Model file for the job. Use its own axes, mm. A direction names the side the tool comes from. Round coordinates to 2 decimals unless told otherwise and drop trailing zeros. Loops run counter-clockwise (first coordinate to the right, second up) from the corner with the lowest first, then second, coordinate; pieces in that order, holes last. Notation, with made-up numbers: M 55,51 L 98,51 A14 ccw 98,69 Z; hole C 17.25,67 d10. An arc over 180 degrees is marked long. Answer in a Markdown table with one row per item.
from build123d import *

# Parameters (mm, degrees)
SKETCH1_W                  = 10
SKETCH1_H                  = 9.1
BASE_FLANGE1_DEPTH         = 0.3
TAB1_DEPTH                 = 0.3
SKETCHED_START             = -12
SKETCHED_BEND1_OUTLINE_W   = 2.75
SKETCHED_BEND1_OUTLINE_H   = 0.3
SKETCHED_BEND1_DEPTH       = 6.725504
SKETCHED_START_2           = -5.274496
SKETCHED_BEND1_2_OUTLINE_W = 2.75
SKETCHED_BEND1_2_OUTLINE_H = 0.3
SKETCHED_BEND1_2_DEPTH     = 0.074434719
SKETCHED_START_3           = -5.35
SKETCHED_BEND1_3_DEPTH     = 0.8
SKETCHED_START_4           = -1.375
SKETCHED_BEND1_4_DEPTH     = 2.75
FILLET1_R                  = 1.5
SKETCH13_R                 = 0.8
CUT_EXTRUDE2_DEPTH         = 13.370499101


with BuildPart() as part:
    # Base-Flange1: sheet metal written as solids
    # Sketch1 → Base-Flange1 (new body)
    with BuildSketch(Plane.XY):
        Rectangle(SKETCH1_W, SKETCH1_H)
    extrude(amount=BASE_FLANGE1_DEPTH)

    # Tab1: sheet metal written as solids
    # Sketch7 → Tab1 (add)
    with BuildSketch(Plane.XY):
        with BuildLine():
            Line((1.375, 0), (1.375, -9.175))
            ThreePointArc((1.375, -9.175), (0, -10.55), (-1.375, -9.175))
            Line((-1.375, -9.175), (-1.375, 0))
            ThreePointArc((-1.375, 0), (0, 1.375), (1.375, 0))
        make_face()
    extrude(amount=TAB1_DEPTH)

    # Sketched Bend1: read off the stored shape, not the designer's step
    # Sketched Bend1 outline → Sketched Bend1 (cut)
    with BuildSketch(Plane(origin=(0, 0, 0), x_dir=(1, 0, 0), z_dir=(0, 1, 0)).offset(SKETCHED_START)):
        with Locations((0, -0.15)):
            Rectangle(SKETCHED_BEND1_OUTLINE_W, SKETCHED_BEND1_OUTLINE_H)
    extrude(amount=SKETCHED_BEND1_DEPTH, mode=Mode.SUBTRACT)

    # Sketched Bend1 2 outline → Sketched Bend1 2 (cut)
    with BuildSketch(Plane(origin=(0, 0, 0), x_dir=(1, 0, 0), z_dir=(0, 1, 0)).offset(SKETCHED_START_2)):
        with Locations((0, -0.15)):
            Rectangle(SKETCHED_BEND1_2_OUTLINE_W, SKETCHED_BEND1_2_OUTLINE_H)
    extrude(amount=SKETCHED_BEND1_2_DEPTH, mode=Mode.SUBTRACT)

    # Sketched Bend1 3 outline → Sketched Bend1 3 (add)
    with BuildSketch(Plane(origin=(0, 0, 0), x_dir=(1, 0, 0), z_dir=(0, 1, 0)).offset(SKETCHED_START_3)):
        with BuildLine():
            Line((-1.375, 4.103982388), (-1.375, 0))
            Line((-1.375, 0), (1.375, 0))
            Line((1.375, 0), (1.375, 4.103982388))
            ThreePointArc((1.375, 4.103982388), (0, 5.478982388), (-1.375, 4.103982388))
        make_face()
    extrude(amount=SKETCHED_BEND1_3_DEPTH)

    # Sketched Bend1 4 outline → Sketched Bend1 4 (cut)
    with BuildSketch(Plane.YZ.offset(SKETCHED_START_4)):
        with BuildLine():
            Line((-5.05, -0.5), (-5.05, -7))
            Line((-5.05, -7), (-4.55, -7))
            Line((-4.55, -7), (-4.55, 0))
            ThreePointArc((-4.55, 0), (-4.903553391, -0.146446609), (-5.05, -0.5))
        make_face()
        with BuildLine():
            Line((-7, -7), (-5.349999999, -7))
            Line((-5.349999999, -7), (-5.35, -0.5))
            ThreePointArc((-5.35, -0.5), (-5.115685425, 0.065685425), (-4.55, 0.3))
            Line((-4.55, 0.3), (-3, 0.3))
            Line((-3, 0.3), (-3, 2))
            Line((-3, 2), (-5.200061281, 2))
            Line((-5.200061281, 2), (-5.200061281, 0))
            Line((-5.200061281, 0), (-7, 0))
            Line((-7, 0), (-7, -7))
        make_face()
    extrude(amount=SKETCHED_BEND1_4_DEPTH, mode=Mode.SUBTRACT)

    # Fillet1
    fillet1_edges = [part.edges().sort_by_distance(p)[0] for p in [
        (-5, 4.55, 0.15),
        (5, 4.55, 0.15),
        (5, -4.55, 0.15),
        (-5, -4.55, 0.15),
    ]]
    fillet(fillet1_edges, radius=FILLET1_R)

    # Sketch13 → Cut-Extrude2 (cut, through all)
    with BuildSketch(Plane.XZ.offset(5.35)):
        with Locations(Location((0, -4.103982388, 0), (0, 0, 270))):
            Circle(SKETCH13_R)
    extrude(amount=-CUT_EXTRUDE2_DEPTH, mode=Mode.SUBTRACT)

    # Sketch14 → Revolve1 (revolve)
    with BuildSketch(Plane(origin=(0, 0, 0), x_dir=(1, 0, 0), z_dir=(0, 1, 0)), mode=Mode.PRIVATE) as revolve1_sk:
        Polygon((0, -0.3), (3.05, -0.3), (1.55, -1.7), (0, -1.7), align=None)
    revolve(revolve1_sk.sketch.rotate(Axis((0, 0, -88.99), (0, 0, 1)), 180), axis=Axis((0, 0, -88.99), (0, 0, 1)))


solid = part.part
1. Saw through at D-D (z = -1.75). Write the cut outline in (x, y) (3 decimals).
Verdict:
| item | result |
|---|---|
| outline | M -1.375,-5.35 L 1.375,-5.35 L 1.375,-5.05 L -1.375,-5.05 Z |
2. Saw through at C-C (z = 1). Write the cut outline in (x, y).
Verdict:
| item | result |
|---|---|
| outline | C 0,0 d4.6 |
3. Saw through at B-B (y = 0). Write the cut outline in (x, z).
Verdict:
| item | result |
|---|---|
| outline | M -5,0 L 5,0 L 5,0.3 L 3.05,0.3 L 1.55,1.7 L -1.55,1.7 L -3.05,0.3 L -5,0.3 Z |
4. Wall check: probe 1 along Z at (x, y) = (-3.5, -3.25); probe 2 along Y at (x, z) = (-0.5, -2); probe 3 along Y at (x, z) = (1.75, 0.25). Give the ranges that are in metal, low to high.
Verdict:
| item | result |
|---|---|
| probe 1 | z = 0 to 0.3 |
| probe 2 | y = -5.35 to -5.05 |
| probe 3 | y = -4.55 to 4.55 |
5. Pin check, flat tips, straight feed: pin 1 (4.5 mm diameter, centred on x = 2, y = 1, fed in from -Z); pin 2 (3 mm diameter, centred on x = 1, z = 1, fed in from -Y); pin 3 (3 mm diameter, centred on x = 0, z = -2.5, fed in from +Y); pin 4 (0.6 mm diameter, centred on y = -5, z = -2, fed in from -X) (3 decimals). Stop position of each tip, or through.
Verdict:
| item | result |
|---|---|
| pin 1 | stops at z = 0 |
| pin 2 | stops at y = -5.35 |
| pin 3 | stops at y = -5.05 |
| pin 4 | stops at x = -1.375 |
6. Mould opens along Z. For faces 4 (the flat face through (0, 0, 1.7)), 5 (the flat face through (0, 0, 0)), 6 (the flat face through (0, -5.35, -2)), 7 (the cylindrical face through (-0.78, -5.2, -3.93)) say: +Z half, -Z half, draft (parallel to the pull), parting line (faces both ways), or undercut.
Verdict:
| item | result |
|---|---|
| face 4 | +Z half |
| face 5 | -Z half |
| face 6 | draft |
| face 7 | undercut |
7. Tool access for faces 1 (the flat face through (-1.2, 3.1, 0.3)), 2 (the cylindrical face through (0.03, -5.2, -5.48)), 3 (the flat face through (0, -5.05, -2)): list every direction of +Z, -Z, +X, -X, +Y, -Y with a clear straight run to the whole face (end or side of a thin tool).
Verdict:
| item | result |
|---|---|
| face 1 | +Z |
| face 2 | -Z, +Y, -Y |
| face 3 | -Z, +X, -X, +Y |
8. Saw through at A-A (x = 0). Write the cut outline in (y, z).
Verdict:
| item | result |
|---|---|
| outline | M -5.35,-5.48 L -5.05,-5.48 L -5.05,-4.9 L -5.35,-4.9 Z; M -5.35,-3.3 L -5.05,-3.3 L -5.05,-0.5 A0.5 cw -4.55,0 L 4.55,0 L 4.55,0.3 L 3.05,0.3 L 1.55,1.7 L -1.55,1.7 L -3.05,0.3 L -4.55,0.3 A0.8 ccw -5.35,-0.5 Z |
